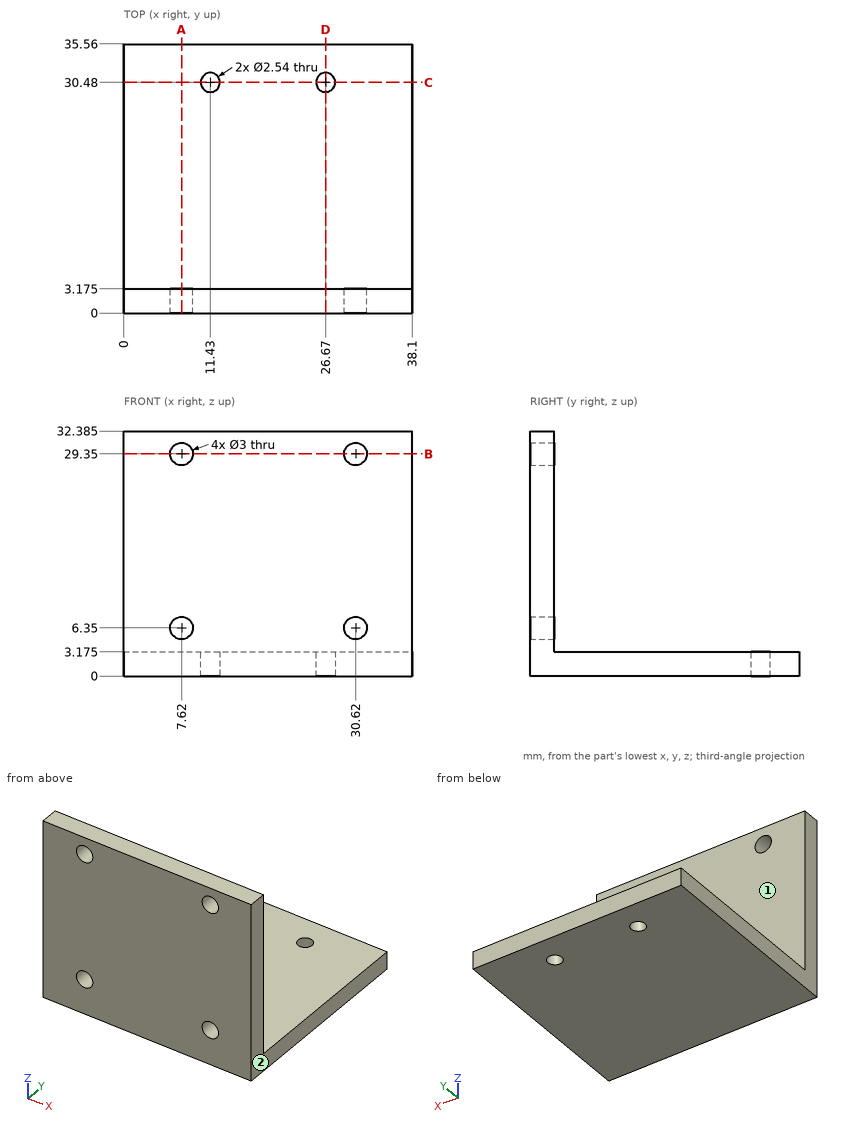
Input: dimensioned drawing with shaded views. Units: mm. Origin: part minimum x, y, z. A direction names the side the tool comes from. Give positions to 0.01 mm unless a question says otherwise; leave off trailing zeros. Loops run counter-clockwise (first coordinate to the right, second up) from the corner with the lowest first, then second, coordinate; pieces in that order, holes last. Notation, with made-up numbers: (27.5, 31) -> (66.5, 31) arc R21 ccw to (66.5, 62) -> close; hole circle Ø11 at (29.5, 60). An arc over 180 degrees is marked (long way). Return JSON: item names as keys, results as strings.
Item 1: Access query for the marked faces 1 and 2. Directions: +Z, -Z, +X, -X, +Y, -Y. A direction counts if a zero-diameter tool reaches every point of the face in a straight line with its end or side. Return the directions, or none.
Filled in:
{"face 1": "+Z, +X, -X, +Y", "face 2": "+Z, -Z, +X, +Y, -Y"}
Item 2: Section A-A, the plane x = 7.62. Output: boundary loops of the cut face in (y, z) (3 decimals), plus the area to 3 significant figures.
Filled in:
{"outline": "(0, 0) -> (35.56, 0) -> (35.56, 3.175) -> (3.175, 3.175) -> (3.175, 4.85) -> (0, 4.85) -> close; (0, 7.85) -> (3.175, 7.85) -> (3.175, 27.85) -> (0, 27.85) -> close; (0, 30.85) -> (3.175, 30.85) -> (3.175, 32.385) -> (0, 32.385) -> close", "area": "187 mm^2"}
Item 3: Section D-D, the plane x = 26.67. Output: boundary loops of the cut face in (y, z) (3 decimals), plus the area to 3 significant figures.
Filled in:
{"outline": "(0, 0) -> (29.21, 0) -> (29.21, 3.175) -> (3.175, 3.175) -> (3.175, 32.385) -> (0, 32.385) -> close; (31.75, 0) -> (35.56, 0) -> (35.56, 3.175) -> (31.75, 3.175) -> close", "area": "198 mm^2"}
Item 4: Section C-C, the plane y = 30.48. Output: boundary loops of the cut face in (x, z) (3 decimals).
Filled in:
{"outline": "(0, 0) -> (10.16, 0) -> (10.16, 3.175) -> (0, 3.175) -> close; (12.7, 0) -> (25.4, 0) -> (25.4, 3.175) -> (12.7, 3.175) -> close; (27.94, 0) -> (38.1, 0) -> (38.1, 3.175) -> (27.94, 3.175) -> close"}
Item 5: Section B-B, the plane z = 29.35. Output: boundary loops of the cut face in (x, y) (3 decimals), plus the area to 3 significant figures.
Filled in:
{"outline": "(0, 0) -> (6.12, 0) -> (6.12, 3.175) -> (0, 3.175) -> close; (9.12, 0) -> (29.12, 0) -> (29.12, 3.175) -> (9.12, 3.175) -> close; (32.12, 0) -> (38.1, 0) -> (38.1, 3.175) -> (32.12, 3.175) -> close", "area": "102 mm^2"}
Item 6: Line query: line 1 (X direction, y = 30.48, z = 1.2); line 2 (Y direction, x = 26.67, z = 0.75); line 3 (Z direction, x = 30, y = 2) (3 decimals). Output: solid intervals per line, ascending.
Filled in:
{"line 1": "0 to 10.16, 12.7 to 25.4, 27.94 to 38.1", "line 2": "0 to 29.21, 31.75 to 35.56", "line 3": "0 to 4.984, 7.716 to 27.984, 30.716 to 32.385"}
Item 7: Pin query (flat end, axial travel): P1, Ø1.5, axis at x = 13.5, z = 5, coming from the +Y side (3 decimals); P2, Ø8, axis at x = 9.5, y = 5.5, coming from the -Z side; P3, Ø2.5, axis at x = 30.62, z = 6.35, coming from the +Y side. Return the tip coordinate at first contact, or that it passes through.
Filled in:
{"P1": "y = 3.175", "P2": "z = 0", "P3": "through"}
